Geometry: final body of the model. Coordinates: model frame, mm. A direction names the side the tool comes from. Coordinates: 2 decimals unless noted, no trailing zeros. Write each loop counter-clockwise with the first axis right and the second up, starting at its lowest first coordinate (ties: lowest second). Pieces come first, ordered by that corner, then holes. Notation, with made-up numbers: (35, -25) - (52, -25) arc R21 cw to (52, 8) - close; hole circle Ø2 at (-16.75, 77). An arc over 180 degrees is marked (long way). Answer as a JSON object with one key per item and string values. Group by question number.
Item 1: First-contact query: pin 1 Ø1.9 at (x, y) = (-12.5, 36.5) entering from +Z; pin 2 Ø1.9 at (y, z) = (26.5, 13) entering from -X; pin 3 Ø1.9 at (y, z) = (60.5, -12) entering from +X; pin 4 Ø4 at (x, z) = (5.5, -9) entering from -Y. Flat tips, straight axial feed; report the tip coordinate or a pass-through.
Item 2: Section C-C on y = -116.5. State how many separate pieces and enclosed holes the cut face has, and give its area (3 significant figures).
Item 3: Section B-B on x = -1. Return loops of the section in (y, z).
Item 4: Line query: line 1 along X through (y, z) = (-57, -22) (3 decimals); line 2 along X through (y, z) = (52, 11.5). Output: solid intervals per line, ascending. Write a range as from..to.
Item 5: Set-up query: faces 4 (the flat face through (-15.875, -2, 22)), 5 (the flat face through (18.651, -2, -13)), 6 (the flat face through (-19.05, -2, 13)), 7 (the flat face through (-6, -152.4, 12)), 8 (the flat face through (-15.875, -2, -22)). Return all of +Z, -Z, +X, -X, +Y, -Y with unobstructed straight access to the full face (end or side cutting, diameter ignored); none if empty.
Item 6: Section A-A on z = 0. Return loops of the section in (x, y).
Item 7: Mould query, pull axis Z, two halves, no side actions, for faces 1 (the flat face through (21, -2, -25.4)), 2 (the flat face through (-22, -2, -15.875)), 3 (the flat face through (15.875, -2, -22)). Classes: pulls with the +Z half, pulls with the -Z half, needs draft (parallel to the pull), parting line crosses it, or undercut.
```python
from build123d import *

# Parameters (mm, degrees)
F0_R     = 2.6035
F0_R_2   = 12.7
F1_DEPTH = 152.4


with BuildPart() as f1:
    # F0 (on Front) → F1 (new body, symmetric)
    with BuildSketch(Plane.XZ):
        Polygon((15.875, -25.4), (25.4, -25.4), (25.4, -15.875), (18.651077, -15.875), (18.651077, -9.525), (25.4, -9.525), (25.4, 9.525), (19.05, 9.525), (19.05, 15.875), (25.4, 15.875), (25.4, 25.4), (15.875, 25.4), (15.875, 19.05), (9.525, 19.05), (9.525, 25.4), (-9.525, 25.4), (-9.525, 19.05), (-15.875, 19.05), (-15.875, 25.4), (-25.4, 25.4), (-25.4, 15.875), (-19.05, 15.875), (-19.05, 9.525), (-25.4, 9.525), (-25.4, -9.525), (-19.05, -9.525), (-19.05, -15.875), (-25.4, -15.875), (-25.4, -25.4), (-15.875, -25.4), (-15.875, -19.05), (-9.525, -19.05), (-9.525, -25.4), (9.525, -25.4), (9.525, -19.05), (15.875, -19.05), align=None)
        with Locations((-12.7, -12.7)):
            Circle(F0_R, mode=Mode.SUBTRACT)
        Circle(F0_R_2, mode=Mode.SUBTRACT)
        with Locations((12.7, -12.7)):
            Circle(F0_R, mode=Mode.SUBTRACT)
        with Locations((-12.7, 12.7)):
            Circle(F0_R, mode=Mode.SUBTRACT)
        with Locations((12.7, 12.7)):
            Circle(F0_R, mode=Mode.SUBTRACT)
    extrude(amount=F1_DEPTH, both=True)


solid = f1.part
```
Checks:
{
 "1": {"pin 1": "z = 19.05", "pin 2": "x = -19.05", "pin 3": "x = 18.65", "pin 4": "through"},
 "2": {"separate pieces": "1", "enclosed holes": "5", "area": "1,660 mm^2"},
 "3": {"outline": "(-152.4, -25.4) - (152.4, -25.4) - (152.4, -12.66) - (-152.4, -12.66) - close; (-152.4, 12.66) - (152.4, 12.66) - (152.4, 25.4) - (-152.4, 25.4) - close"},
 "4": {"line 1": "-25.4..-15.875, -9.525..9.525, 15.875..25.4", "line 2": "-19.05..-15.01, -10.39..-5.39, 5.39..10.39, 15.01..19.05"},
 "5": {"face 4": "+Z, +Y, -Y", "face 5": "+X, +Y, -Y", "face 6": "-X, +Y, -Y", "face 7": "+Z, -Z, +X, -X, -Y", "face 8": "-Z, +Y, -Y"},
 "6": {"outline": "(-25.4, -152.4) - (-12.7, -152.4) - (-12.7, 152.4) - (-25.4, 152.4) - close; (12.7, -152.4) - (25.4, -152.4) - (25.4, 152.4) - (12.7, 152.4) - close"},
 "7": {"face 1": "pulls with the -Z half", "face 2": "undercut", "face 3": "needs draft"}
}
